Here's how the part is built. I have some questions about the finished solid (model axes, mm). A direction names the side the tool comes from. Round coordinates to 2 decimals unless told otherwise and drop trailing zeros. Loops run counter-clockwise (first coordinate to the right, second up) from the corner with the lowest first, then second, coordinate; pieces in that order, holes last. Notation, with made-up numbers: (7.25, 46) - (46.25, 46) arc R33 cw to (46.25, 80) - close; hole circle Ø2 at (16.5, 4.25). An arc over 180 degrees is marked (long way). Answer as a JSON object with one key per item and string values. Group by question number.
1) If we mould it in two halves opening along X, with no side actions, what happens to faces 1 (the face through (-11, 13, 0)), 2 (the face through (-14.9, 7.4, 3.81)), 3 (the face through (-3.903, 17.576, 3.397))? For each: pulls with the +X half, pulls with the -X half, needs draft (parallel to the pull), parting line crosses it, or undercut.
2) Will these pins go through, and if not, where does the flat tip stop? P1, Ø14, axis at x = 0, y = 0, coming from the -Z side; P2, Ø4, axis at x = 2, z = 2, coming from the -Y side; P3, Ø2, axis at y = 11, z = 5, coming from the +X side; P4, Ø4.5, axis at x = -0.5, y = 1.5, coming from the -Z side.
3) I want a section at C-C, the plane z = 2.5. Please give me the cut outline in (x, y) (1 decimal), then the cut area to 3 significant figures.
4) Which directions (+Z, -Z, +X, -X, +Y, -Y) give clear straight access to the entire face, cutting with the end or side of a thin tool? Please do faces 4 (the face through (-3.4, 3.4, 0)), 5 (the face through (1, 2, 3.81)).
5) If I drill on line 1 along Y through (x, z) = (-4, 1.75); line 2 along Y through (x, z) = (0, 5.35); line 3 along X through (y, z) = (0, 1.85) (1 decimal), over which ranges is the centre line in solid material (lowest first)? Write a range as [from, to].
6) I want a section at D-D, the plane z = 6.25. Please give me the cut outline in (x, y), then the cut area to 3 significant figures.
from build123d import *

# Parameters (mm, degrees)
F3_D     = 3.7973
F4_R     = 4.445
F4_R_2   = 1.89865
F5_DEPTH = 3.81
F6_R     = 1.27


with BuildPart() as f1:
    # F0 (on Front) → F1 (revolve)
    with BuildSketch(Plane.XZ):
        Polygon((17.9125677648, 6.731), (0, 6.731), (0, 0), (16.4465, 0), (16.4465, 3.81), (16.8275, 3.81), (16.8275, 0), (18.0975, 0), align=None)
    revolve(axis=Axis((0, 0, 3.3655), (0, 0, -1)))

    # F3 (through all)
    with Locations(Plane.XY.offset(6.731)):
        with Locations((0, 0)):
            Hole(F3_D / 2)

    # F4 (on face) → F5 (cut)
    with BuildSketch(Plane(origin=(0, 0, 0), x_dir=(1, 0, 0), z_dir=(0, 0, -1))):
        Circle(F4_R)
        Circle(F4_R_2, mode=Mode.SUBTRACT)
    extrude(amount=-F5_DEPTH, mode=Mode.SUBTRACT)

    # F6
    f6_edges = [f1.edges().sort_by_distance(p)[0] for p in [
        (-17.912568, 0, 6.731),
    ]]
    fillet(f6_edges, radius=F6_R)


solid = f1.part
Outcome:
{
 "1": {"face 1": "needs draft", "face 2": "undercut", "face 3": "parting line crosses it"},
 "2": {"P1": "z = 0", "P2": "y = -18.07", "P3": "x = 14.92", "P4": "z = 3.81"},
 "3": {"outline": "circle Ø36.1 at (0, 0); circle Ø32.9 at (0, 0); hole circle Ø33.7 at (0, 0); hole circle Ø8.9 at (0, 0)", "area": "919 mm^2"},
 "4": {"face 4": "-Z, +X, -X, +Y, -Y", "face 5": "-Z"},
 "5": {"line 1": "[-17.6, -16.35], [-15.95, -1.94], [1.94, 15.95], [16.35, 17.6]", "line 2": "[-17.95, -1.9], [1.9, 17.95]", "line 3": "[-18, -16.8], [-16.4, -4.4], [4.4, 16.4], [16.8, 18]"},
 "6": {"outline": "circle Ø35.34 at (0, 0); hole circle Ø3.8 at (0, 0)", "area": "970 mm^2"}
}
